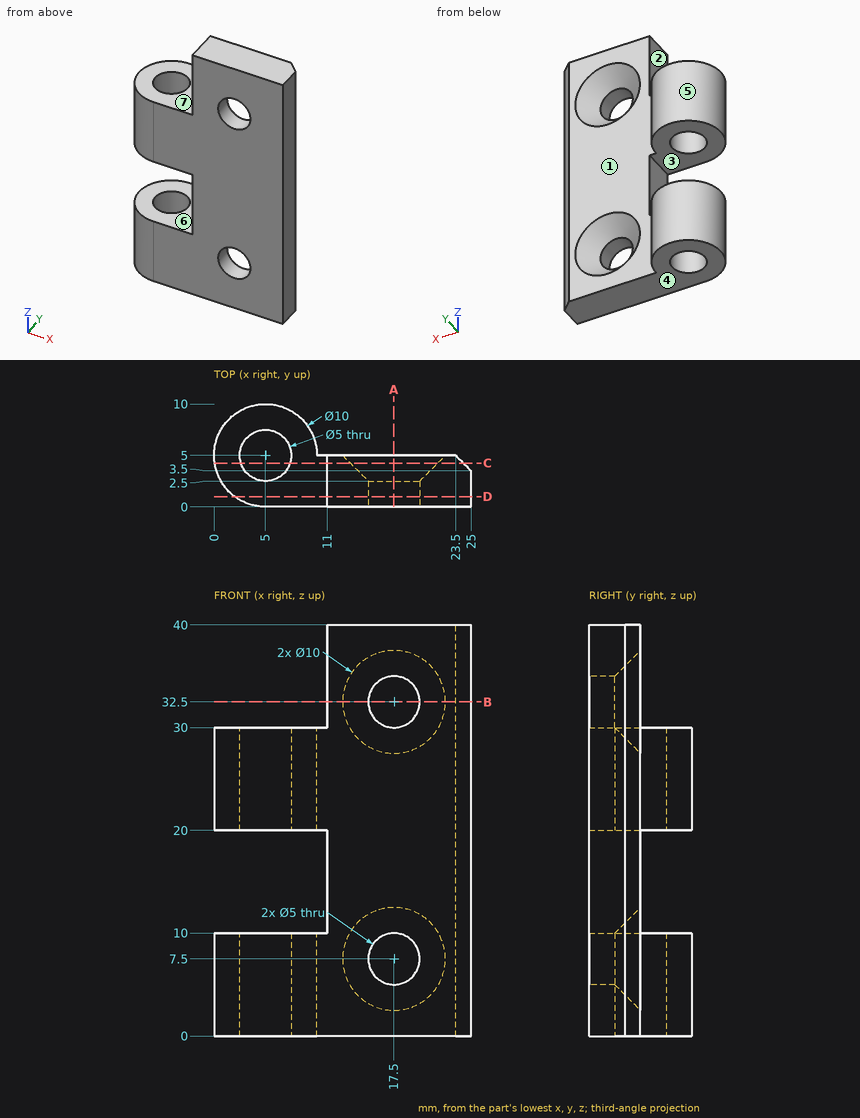
Geometry check sheet. Reference: drawing and pictorial views, mm from the part's lowest x, y, z. A direction names the side the tool comes from. Coordinates: 2 decimals unless noted, no trailing zeros. Order: outer loops, then holes, each group sorted by start corner. A loop starts at its lowest first (then second) coordinate and runs counter-clockwise, first axis right, second up.
Item 1: Mould release check, pull along Z, two halves, no side actions. Record for the marked faces 4, 5, 6 and 7: released by +Z, released by -Z, zero draft, split by the parting line, or undercut.
Item 2: Section check A-A (x = 17.5). Enter the section's corners in (y, z).
Item 3: Section check D-D (y = 1). Enter the section's corners in (x, z).
Item 4: Depth check by flat-ended pin: pin 1 (4 mm diameter, centred on x = 15, z = 22.5, fed in from +Y); pin 2 (1 mm diameter, centred on y = 3, z = 5.5, fed in from -X); pin 3 (4 mm diameter, centred on y = 1.5, z = 33.5, fed in from -X). Enter the tip coordinate at first touch or a pass-through.
Item 5: Scan lines: line 1 along Z through (x, y) = (17.5, 1.4); line 2 along Z through (x, y) = (7.25, 0.75); line 3 along X through (y, z) = (1.9, 32.5). Record each from-to range of solid material in increasing order.
Item 6: Tool access check on the marked faces 1, 2 and 3. Record the directions out of +Z, -Z, +X, -X, +Y, -Y that give a thin tool (end or side, any length) a straight path to the whole face; none if there is none.
Item 7: Section check B-B (z = 32.5). Enter the section's corners in (x, y).
Item 8: Section check C-C (y = 4.25). Enter the section's corners in (x, z).
Check sheet entries:
1. face 4: released by -Z
1. face 5: zero draft
1. face 6: undercut
1. face 7: released by +Z
2. outline: (0, 0) - (5, 0) - (5, 2.5) - (2.5, 5) - (0, 5) - close; (0, 10) - (2.5, 10) - (5, 12.5) - (5, 27.5) - (2.5, 30) - (0, 30) - close; (0, 35) - (2.5, 35) - (5, 37.5) - (5, 40) - (0, 40) - close
3. outline: (2, 0) - (25, 0) - (25, 40) - (11, 40) - (11, 30) - (2, 30) - (2, 20) - (11, 20) - (11, 10) - (2, 10) - close; hole circle Ø5 at (17.5, 7.5); hole circle Ø5 at (17.5, 32.5)
4. pin 1: stops at y = 5
4. pin 2: stops at x = 0.23
4. pin 3: stops at x = 11
5. line 1: z = 0 to 5, 10 to 30, 35 to 40
5. line 2: z = 0 to 10, 20 to 30
5. line 3: x = 11 to 15, 20 to 25
6. face 1: +Z, -Z, +X, +Y
6. face 2: +Z, -X, +Y, -Y
6. face 3: -X, +Y, -Y
7. outline: (11, 0) - (15, 0) - (15, 2.5) - (12.5, 5) - (11, 5) - close; (20, 0) - (25, 0) - (25, 3.5) - (23.5, 5) - (22.5, 5) - (20, 2.5) - close
8. outline: (0.06, 0) - (2.62, 0) - (2.62, 10) - (0.06, 10) - close; (0.06, 20) - (2.62, 20) - (2.62, 30) - (0.06, 30) - close; (7.38, 0) - (24.25, 0) - (24.25, 40) - (11, 40) - (11, 30) - (7.38, 30) - (7.38, 20) - (11, 20) - (11, 10) - (7.38, 10) - close; hole circle Ø8.5 at (17.5, 7.5); hole circle Ø8.5 at (17.5, 32.5)
